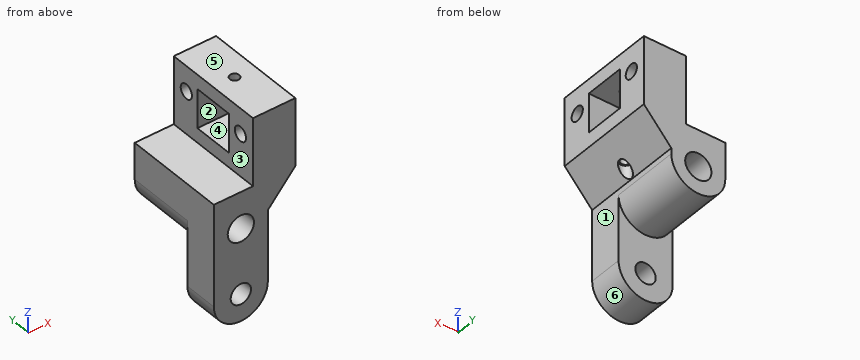
from build123d import *

# Parameters (mm, degrees)
SKETCH_1_R          = 6
SKETCH_1_R_2        = 7.75
EXTRUDE_1_DEPTH     = 60
CUT_EXTRUDE_START   = -40
SKETCH_3_R          = 15.93293451
CUT_EXTRUDE_1_DEPTH = 40
CUT_EXTRUDE_2_DEPTH = 40
SKETCH_5_R          = 4.25
CUT_EXTRUDE_3_DEPTH = 108.890486757
SKETCH_6_W          = 30
SKETCH_6_H          = 60
SKETCH_6_R          = 4.25
EXTRUDE_2_DEPTH     = 30
SKETCH_8_W          = 30
SKETCH_8_H          = 60
CUT_EXTRUDE_4_DEPTH = 30
SKETCH_10_W         = 31.86586902
SKETCH_10_H         = 40
CUT_EXTRUDE_6_DEPTH = 110
SKETCH_13_W         = 25
SKETCH_13_H         = 60
EXTRUDE_4_DEPTH     = 40
EXTRUDE_5_DEPTH     = 60
SKETCH_15_R         = 4.25
SKETCH_15_W         = 23
SKETCH_15_H         = 23.812373312
CUT_EXTRUDE_7_DEPTH = 107.065656667
SKETCH_16_R         = 2.75
CUT_EXTRUDE_8_DEPTH = 252.064107028
SKETCH_17_R         = 3.5
CUT_EXTRUDE_9_DEPTH = 60


with BuildPart() as part:
    # 草图1 → 凸台-拉伸1 (new body)
    with BuildSketch(Plane(origin=(0, 0, 0), x_dir=(1, 0, 0), z_dir=(0, 1, 0))):
        with BuildLine():
            Line((74.517406475, 16.185183146), (74.517406475, -83.814816854))
            Line((74.517406475, -83.814816854), (106.383275494, -83.814816854))
            Line((106.383275494, -83.814816854), (106.383275494, 16.185183146))
            ThreePointArc((106.383275494, 16.185183146), (90.450340985, 32.118117656), (74.517406475, 16.185183146))
        make_face()
        with Locations(Location((90.450340985, 16.185183146, 0), (0, 0, 270))):
            Circle(SKETCH_1_R, mode=Mode.SUBTRACT)
        with Locations(Location((90.450340985, -22.314816854, 0), (0, 0, 270))):
            Circle(SKETCH_1_R_2, mode=Mode.SUBTRACT)
    extrude(amount=EXTRUDE_1_DEPTH)

    # 草图3 → 切除-拉伸1 (cut)
    with BuildSketch(Plane(origin=(0, 60, 0), x_dir=(1, 0, 0), z_dir=(0, 1, 0)).offset(CUT_EXTRUDE_START)):
        with Locations((90.450340985, 16.185183146)):
            Circle(SKETCH_3_R)
    extrude(amount=CUT_EXTRUDE_1_DEPTH, mode=Mode.SUBTRACT)

    # 草图4 → 切除-拉伸2 (cut)
    with BuildSketch(Plane(origin=(0, 60, 0), x_dir=(1, 0, 0), z_dir=(0, 1, 0))):
        with BuildLine():
            Line((74.517406475, 16.185183146), (74.517406475, -22.314816854))
            ThreePointArc((74.517406475, -22.314816854), (90.450340985, -6.381882344), (106.383275494, -22.314816854))
            Line((106.383275494, -22.314816854), (106.383275494, 16.185183146))
            Line((106.383275494, 16.185183146), (74.517406475, 16.185183146))
        make_face()
    extrude(amount=-CUT_EXTRUDE_2_DEPTH, mode=Mode.SUBTRACT)

    # 草图5 → 切除-拉伸3 (cut, through all)
    with BuildSketch(Plane.ZY.offset(-74.517406475)):
        with Locations((68.814816854, 9.5)):
            Circle(SKETCH_5_R)
        with Locations((68.814816854, 50.5)):
            Circle(SKETCH_5_R)
    extrude(amount=-CUT_EXTRUDE_3_DEPTH, mode=Mode.SUBTRACT)

    # 草图6 → 凸台-拉伸2 (add)
    with BuildSketch(Plane(origin=(106.383275494, 0, 0), x_dir=(0, 0, -1), z_dir=(1, 0, 0))):
        with Locations((-68.814816854, 30)):
            Rectangle(SKETCH_6_W, SKETCH_6_H)
        with Locations(Location((-68.814816854, 50.5, 0), (0, 0, 180))):
            Circle(SKETCH_6_R, mode=Mode.SUBTRACT)
        with Locations(Location((-68.814816854, 9.5, 0), (0, 0, 180))):
            Circle(SKETCH_6_R, mode=Mode.SUBTRACT)
    extrude(amount=EXTRUDE_2_DEPTH)


with BuildPart() as body_2:
    # 镜向1: mirrored copy
    add(part.part.mirror(Plane.ZY.offset(-136.383275494)))

    # 草图8 → 切除-拉伸4 (cut)
    with BuildSketch(Plane.ZY.offset(-136.383275494)):
        with Locations((68.814816854, 30)):
            Rectangle(SKETCH_8_W, SKETCH_8_H)
    extrude(amount=-CUT_EXTRUDE_4_DEPTH, mode=Mode.SUBTRACT)

    # 草图10 → 切除-拉伸6 (cut)
    with BuildSketch(Plane(origin=(0, 60, 0), x_dir=(1, 0, 0), z_dir=(0, 1, 0))):
        with Locations((182.316210004, -63.814816854)):
            Rectangle(SKETCH_10_W, SKETCH_10_H)
    extrude(amount=-CUT_EXTRUDE_6_DEPTH, mode=Mode.SUBTRACT)

    # 草图13 → 凸台-拉伸4 (add)
    with BuildSketch(Plane.XY.offset(43.814816854)):
        with Locations((201.95918151, 30)):
            Rectangle(SKETCH_13_W, SKETCH_13_H)
    extrude(amount=EXTRUDE_4_DEPTH)

    # 草图14 → 凸台-拉伸5 (add)
    with BuildSketch(Plane(origin=(0, 60, 0), x_dir=(1, 0, 0), z_dir=(0, 1, 0))):
        Polygon((214.45918151, -43.814816854), (198.249144514, -43.814816854), (198.249144514, -25.604816854), align=None)
    extrude(amount=-EXTRUDE_5_DEPTH)

    # 草图15 → 切除-拉伸7 (cut, through all)
    with BuildSketch(Plane.ZY.offset(-189.45918151)):
        with Locations((68.814816854, 9.5)):
            Circle(SKETCH_15_R)
        with Locations((68.814816854, 50.5)):
            Circle(SKETCH_15_R)
        with Locations((63.87118854, 30.184894764)):
            Rectangle(SKETCH_15_W, SKETCH_15_H)
    extrude(amount=-CUT_EXTRUDE_7_DEPTH, mode=Mode.SUBTRACT)

    # 草图16 → 切除-拉伸8 (cut, through all)
    with BuildSketch(Plane.XY.offset(83.814816854)):
        with Locations((201.95918151, 30)):
            Circle(SKETCH_16_R)
    extrude(amount=-CUT_EXTRUDE_8_DEPTH, mode=Mode.SUBTRACT)

    # 草图17 → 切除-拉伸9 (cut)
    with BuildSketch(Plane.XY.offset(34.37118854)):
        with Locations((201.95918151, 30)):
            Circle(SKETCH_17_R)
    extrude(amount=-CUT_EXTRUDE_9_DEPTH, mode=Mode.SUBTRACT)


solid = body_2.part
Read the model definition and answer for the solid it produces. Units are mm, in the model's axes. Face numbers are marked on the shaded views. A direction names the side the tool comes from. Coordinates: 2 decimals unless noted, no trailing zeros. Loops run counter-clockwise (first coordinate to the right, second up) from the corner with the lowest first, then second, coordinate; pieces in that order, holes last.
Q1. Each of these flat-tipped pins is pushed along its axis until it touches: pin 1 Ø11 at (x, y) = (201.96, 30) entering from +Z; pin 2 Ø5 at (y, z) = (50.5, 68.81) entering from -X; pin 3 Ø7 at (x, y) = (176, 40.5) entering from +Z; pin 4 Ø1.5 at (x, y) = (172, 43) entering from -Z. Where does it stop, or does it pass through?
Q2. The mould has two halves that part along Z. Classify the marked faces 4, 5 and 6: +Z half, -Z half, draft (parallel to the pull), parting line (faces both ways), or undercut.
Q3. The part is cut by section D-D on x = 186. Write down the section's boundary in (y, z).
Q4. Which of the six approach directions +Z, -Z, +X, -X, +Y, -Y give full straight-line access (tool end or side, diameter ignored) to the marked faces 1, 2 and 3?
Q5. The part is cut by section C-C on y = 9.5. Write down the section's boundary in (x, z).
Q6. The part is cut by section B-B on y = 50.5. Write down the section's boundary in (x, z), and give its area (3 significant figures).
Q7. Consider probe 1 along Y at (x, z) = (212.5, 71.5); probe 2 along Z at (x, y) = (187.5, 16); probe 3 along Y at (x, z) = (195.5, -5.5). Determine where each line is inside the solid, lowest interval first.
Q8. The part is cut by section A-A on z = 62.5. Write down the section's boundary in (x, y).
Results below:
1. pin 1: stops at z = 83.81
1. pin 2: passes through
1. pin 3: stops at z = 43.81
1. pin 4: stops at z = 9.57
2. face 4: undercut
2. face 5: +Z half
2. face 6: -Z half
3. outline: (0, -31.69) - (20, -31.69) - (20, -20.92) - (0, -20.92) - close; (0, -11.45) - (20, -11.45) - (20, 6.81) - (60, 6.81) - (60, 15.5) - (0, 15.5) - close; (0, 29.13) - (60, 29.13) - (60, 43.81) - (0, 43.81) - close
4. face 1: -Z, +X, +Y, -Y
4. face 2: +X, -X
4. face 3: +Z, -X, +Y, -Y
5. outline: (166.38, -16.19) arc R15.93 ccw to (198.25, -16.19) - (198.25, 25.6) - (214.46, 43.81) - (214.46, 64.56) - (189.46, 64.56) - (189.46, 43.81) - (166.38, 43.81) - close; (189.46, 73.06) - (214.46, 73.06) - (214.46, 83.81) - (189.46, 83.81) - close; hole circle Ø15.5 at (182.32, 22.31); hole circle Ø12 at (182.32, -16.19)
6. outline: (166.38, 22.31) arc R15.93 ccw to (198.25, 22.31) - (198.25, 25.6) - (214.46, 43.81) - (214.46, 64.56) - (189.46, 64.56) - (189.46, 43.81) - (166.38, 43.81) - close; (189.46, 73.06) - (214.46, 73.06) - (214.46, 83.81) - (189.46, 83.81) - close; hole circle Ø15.5 at (182.32, 22.31)
6. area: 1,830 mm2
7. probe 1: y = 0 to 6.21, 12.79 to 18.28, 42.09 to 47.21, 53.79 to 60
7. probe 2: z = -31.25 to -19.21, -13.16 to 16.55, 28.08 to 43.81
7. probe 3: y = 0 to 20
8. outline: (189.46, 0) - (214.46, 0) - (214.46, 18.28) - (189.46, 18.28) - close; (189.46, 42.09) - (214.46, 42.09) - (214.46, 60) - (189.46, 60) - close
